Source: CAD feature listing. Evaluate the final solid. Frame: model axes, mm. A direction names the side the tool comes from. Round coordinates to 2 decimals unless told otherwise and drop trailing zeros. Order: outer loops, then holes, each group sorted by start corner. A loop starts at its lowest first (then second) coordinate and runs counter-clockwise, first axis right, second up.
```python
from build123d import *

# Parameters (mm, degrees)
BOSS_EXTRUDE1_DEPTH = 70.8
CUT_EXTRUDE1_DEPTH  = 89.971118909
BOSS_EXTRUDE2_DEPTH = 1.976458037


with BuildPart() as part:
    # Sketch1 → Boss-Extrude1 (new body)
    with BuildSketch(Plane.XY):
        with BuildLine():
            Line((2.54, 0), (35.56, 0))
            ThreePointArc((35.56, 0), (37.356051224, -0.743948776), (38.1, -2.54))
            Line((38.1, -2.54), (38.1, -35.56))
            ThreePointArc((38.1, -35.56), (37.356051224, -37.356051224), (35.56, -38.1))
            Line((35.56, -38.1), (2.54, -38.1))
            ThreePointArc((2.54, -38.1), (0.743948776, -37.356051224), (0, -35.56))
            Line((0, -35.56), (0, -2.54))
            ThreePointArc((0, -2.54), (0.743948776, -0.743948776), (2.54, 0))
        make_face()
        with BuildLine():
            Line((5.3086, -2.7686), (32.7914, -2.7686))
            ThreePointArc((32.7914, -2.7686), (34.587451224, -3.512548776), (35.3314, -5.3086))
            Line((35.3314, -5.3086), (35.3314, -32.7914))
            ThreePointArc((35.3314, -32.7914), (34.587451224, -34.587451224), (32.7914, -35.3314))
            Line((32.7914, -35.3314), (5.3086, -35.3314))
            ThreePointArc((5.3086, -35.3314), (3.512548776, -34.587451224), (2.7686, -32.7914))
            Line((2.7686, -32.7914), (2.7686, -5.3086))
            ThreePointArc((2.7686, -5.3086), (3.512548776, -3.512548776), (5.3086, -2.7686))
        make_face(mode=Mode.SUBTRACT)
    extrude(amount=BOSS_EXTRUDE1_DEPTH)

    # Sketch2 → Cut-Extrude1 (cut, through all)
    with BuildSketch(Plane(origin=(38.1, 0, 0), x_dir=(0, 0, -1), z_dir=(1, 0, 0))):
        Polygon((-70.8, 0), (-67.46668192, -38.1), (-70.8, -38.1), align=None)
    extrude(amount=-CUT_EXTRUDE1_DEPTH, mode=Mode.SUBTRACT)

    # Sketch3 → Boss-Extrude2 (add)
    with BuildSketch(Plane(origin=(0, -6.147145489, 70.262194457), x_dir=(1, 0, 0), z_dir=(0, -0.08715574274765149, 0.9961946980917462))):
        with BuildLine():
            Line((2.54, -32.074909224), (35.56, -32.074909224))
            add(Edge.make_bspline(
                [(35.56, -32.074909224), (38.1, -32.074909224), (38.1, -29.525206837)],
                knots=[0, 0, 0, 1.570796327, 1.570796327, 1.570796327], degree=2, weights=[1, 0.707106781, 1]))
            Line((38.1, -29.525206837), (38.1, 3.620924199))
            add(Edge.make_bspline(
                [(38.1, 3.620924199), (38.1, 6.170626587), (35.56, 6.170626587)],
                knots=[1.570796327, 1.570796327, 1.570796327, 3.141592654, 3.141592654, 3.141592654], degree=2, weights=[1, 0.707106781, 1]))
            Line((35.56, 6.170626587), (2.54, 6.170626587))
            add(Edge.make_bspline(
                [(2.54, 6.170626587), (0, 6.170626587), (0, 3.620924199)],
                knots=[3.141592654, 3.141592654, 3.141592654, 4.71238898, 4.71238898, 4.71238898], degree=2, weights=[1, 0.707106781, 1]))
            Line((0, 3.620924199), (0, -29.525206837))
            add(Edge.make_bspline(
                [(0, -29.525206837), (0, -32.074909224), (2.54, -32.074909224)],
                knots=[4.71238898, 4.71238898, 4.71238898, 6.283185307, 6.283185307, 6.283185307], degree=2, weights=[1, 0.707106781, 1]))
        make_face()
    extrude(amount=BOSS_EXTRUDE2_DEPTH)


solid = part.part
```
1. Access query for faces 1 (the face through (0.764, -37.376, 33.371)), 2 (the face through (37.376, -37.336, 33.371)), 3 (the face through (19, -38.1, 33)), 4 (the face through (18.822, -18.822, 69.153)). Directions: +Z, -Z, +X, -X, +Y, -Y. A direction counts if a zero-diameter tool reaches every point of the face in a straight line with its end or side. Return the directions, or none.
2. Section C-C on y = -22. Return loops of the section in (x, z).
3. Line query: line 1 along X through (y, z) = (-14, 49); line 2 along Y through (x, z) = (11, 34); line 3 along Y through (x, z) = (35, 52). Output: solid intervals per line, ascending.
4. Section D-D on y = -11. Return loops of the section in (x, z).
5. Pull-direction query (X, two-part tool) for faces 5 (the face through (0, -19, 34)), 6 (the face through (34.568, -3.493, 34.785)), 7 (the face through (19.281, -0.085, 71.771)); classes: released by +X, released by -X, zero draft, split by the parting line, or undercut.
6. First-contact query: pin 1 (1 mm diameter, centred on x = 7, z = 54, fed in from -Y); pin 2 (4 mm diameter, centred on x = 27, y = -9, fed in from -Z); pin 3 (6 mm diameter, centred on x = 27, y = -5, fed in from +Z). Flat tips, straight axial feed; report the tip coordinate or a pass-through.
7. Section A-A on z = 28. Return loops of the section in (x, y).
8. Section B-B on x = 23.5. Return loops of the section in (y, z).
Result:
1. face 1: -Z, -X, -Y
1. face 2: -Z, +X, -Y
1. face 3: -Z, +X, -X, -Y
1. face 4: -Z
2. outline: (0, 0) - (2.77, 0) - (2.77, 68.88) - (35.33, 68.88) - (35.33, 0) - (38.1, 0) - (38.1, 70.86) - (0, 70.86) - close
3. line 1: x = 0 to 2.77, 35.33 to 38.1
3. line 2: y = -38.1 to -35.33, -2.77 to 0
3. line 3: y = -38.1 to -34.05, -4.05 to 0
4. outline: (0, 0) - (2.77, 0) - (2.77, 69.84) - (35.33, 69.84) - (35.33, 0) - (38.1, 0) - (38.1, 71.82) - (0, 71.82) - close
5. face 5: released by -X
5. face 6: undercut
5. face 7: zero draft
6. pin 1: stops at y = -38.1
6. pin 2: stops at z = 69.84
6. pin 3: stops at z = 72.61
7. outline: (0, -35.56) arc R2.54 ccw to (2.54, -38.1) - (35.56, -38.1) arc R2.54 ccw to (38.1, -35.56) - (38.1, -2.54) arc R2.54 ccw to (35.56, 0) - (2.54, 0) arc R2.54 ccw to (0, -2.54) - close; hole (2.77, -32.79) arc R2.54 ccw to (5.31, -35.33) - (32.79, -35.33) arc R2.54 ccw to (35.33, -32.79) - (35.33, -5.31) arc R2.54 ccw to (32.79, -2.77) - (5.31, -2.77) arc R2.54 ccw to (2.77, -5.31) - close
8. outline: (-38.27, 69.44) - (-38.1, 67.47) - (-38.1, 0) - (-35.33, 0) - (-35.33, 67.71) - (-2.77, 70.56) - (-2.77, 0) - (0, 0) - (0, 70.8) - (-0.17, 72.77) - close
